Check sheet for the modelled part. Datum: model origin and axes. Units: mm. Round coordinates to 2 decimals unless told otherwise and drop trailing zeros. Order: outer loops, then holes, each group sorted by start corner. A loop starts at its lowest first (then second) coordinate and runs counter-clockwise, first axis right, second up.
Q1. Cross-section at B-B on x = 60. Record the cut outline in (y, z), then the cut area to 3 significant figures.
Q2. Cross-section at C-C on z = 30. Record the cut outline in (x, y), then the cut area to 3 significant figures.
Q3. Cross-section at D-D on y = -3. Give the number of separate pieces and of enclosed holes in the cut face, then the cut area to 3 significant figures.
Q4. Mould release check, pull along Y, two halves, no side actions. Record for faces 1 (the flat face through (41, 2, 25)), 2 (the flat face through (35.231, -21.887, 12.325)), 3 (the cylindrical face through (52.507, 0.33, 9.86)): +Y half, -Y half, draft (parallel to the pull), parting line (faces both ways), or undercut.
Q5. Scan lines: probe 1 along Y at (x, z) = (0, 17); probe 2 along X at (y, z) = (-0.5, 28); probe 3 along Y at (x, z) = (-12.5, 43). Record each from-to range of solid material in increasing order.
Q6. Cross-section at A-A on z = 11. Record the cut outline in (x, y), then the cut area to 3 significant figures.
Q7. Depth check by flat-ended pin: P1, Ø24, axis at x = 60, y = 0, coming from the -Z side; P2, Ø2, axis at y = 5.5, z = 37, coming from the +X side; P3, Ø5, axis at x = 60.5, y = 9, coming from the +Z side; P4, Ø5, axis at x = 38.5, y = -21, coming from the +Z side. Enter the tip coordinate at first touch or a pass-through.
from build123d import *

# Parameters (mm, degrees)
F0_R     = 15
F0_R_2   = 7.5
F1_DEPTH = 25
F2_DEPTH = 45
F3_R     = 3
F4_R     = 5


with BuildPart() as f1:
    # F0 (on Top) → F1 (new body)
    with BuildSketch(Plane.XY):
        with BuildLine():
            ThreePointArc((7.5, -29.047375), (23.717082, -18.371173), (30, 0))
            ThreePointArc((30, 0), (23.717082, 18.371173), (7.5, 29.047375))
            ThreePointArc((7.5, 29.047375), (-30, 0), (7.5, -29.047375))
        make_face()
        Circle(F0_R, mode=Mode.SUBTRACT)
        with BuildLine():
            ThreePointArc((7.5, 29.047375), (23.717082, 18.371173), (30, 0))
            ThreePointArc((30, 0), (23.717082, -18.371173), (7.5, -29.047375))
            Line((7.5, -29.047375), (63.75, -14.523688))
            ThreePointArc((63.75, -14.523688), (45, 0), (63.75, 14.523688))
            Line((63.75, 14.523688), (7.5, 29.047375))
        make_face()
        with BuildLine():
            ThreePointArc((75, 0), (71.858541, 9.185587), (63.75, 14.523688))
            ThreePointArc((63.75, 14.523688), (45, 0), (63.75, -14.523688))
            ThreePointArc((63.75, -14.523688), (71.858541, -9.185587), (75, 0))
        make_face()
        with Locations((60, 0)):
            Circle(F0_R_2, mode=Mode.SUBTRACT)
    extrude(amount=F1_DEPTH)

    # F0 (on Top) → F2 (join)
    with BuildSketch(Plane.XY):
        with BuildLine():
            ThreePointArc((7.5, -29.047375), (23.717082, -18.371173), (30, 0))
            ThreePointArc((30, 0), (23.717082, 18.371173), (7.5, 29.047375))
            ThreePointArc((7.5, 29.047375), (-30, 0), (7.5, -29.047375))
        make_face()
        Circle(F0_R, mode=Mode.SUBTRACT)
    extrude(amount=F2_DEPTH)

    # F3
    f3_edges = [f1.edges().sort_by_distance(p)[0] for p in [
        (-7.5, 29.047375, 45),
    ]]
    fillet(f3_edges, radius=F3_R)

    # F4
    f4_edges = [f1.edges().sort_by_distance(p)[0] for p in [
        (-15, 0, 45),
        (52.5, 0, 25),
    ]]
    fillet(f4_edges, radius=F4_R)


solid = f1.part
Results found:
1. outline: (-15.49, 0) - (-7.5, 0) - (-7.5, 20) arc R5 ccw to (-12.5, 25) - (-15.49, 25) - close; (7.5, 0) - (15.49, 0) - (15.49, 25) - (12.5, 25) arc R5 ccw to (7.5, 20) - close
1. area: 389 mm2
2. outline: (7.5, -29.05) arc R30 ccw to (30, 0) arc R30 ccw to (7.5, 29.05) arc R30 ccw (long way) to start; hole circle Ø30 at (0, 0)
2. area: 2,120 mm2
3. separate pieces: 3
3. enclosed holes: 0
3. area: 2,110 mm2
4. face 1: draft
4. face 2: -Y half
4. face 3: undercut
5. probe 1: y = -30 to -15, 15 to 30
5. probe 2: x = -30 to -14.99, 14.99 to 30
5. probe 3: y = -27.08 to -9.99, 9.99 to 27.08
6. outline: (7.5, -29.05) - (63.75, -14.52) arc R15 ccw to (63.75, 14.52) - (7.5, 29.05) arc R30 ccw (long way) to start; hole circle Ø30 at (0, 0); hole circle Ø15 at (60, 0)
6. area: 3,670 mm2
7. P1: stops at z = 0
7. P2: stops at x = 29.66
7. P3: stops at z = 24.9
7. P4: stops at z = 25
